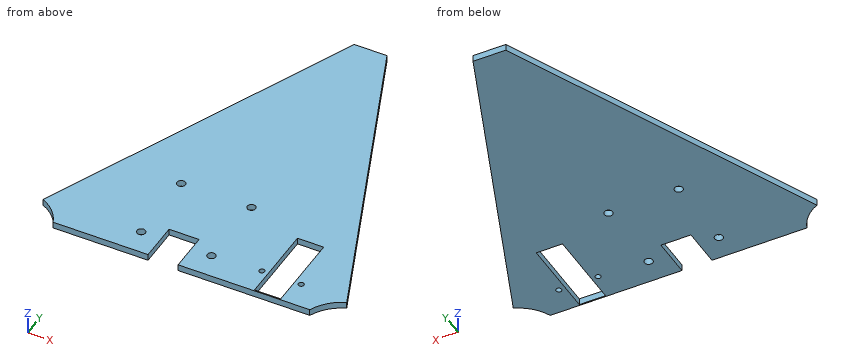
from build123d import *

# Parameters (mm, degrees)
BOSS_EXTRUDE1_DEPTH     = 7.62
SKETCH5_R               = 15.875
CUT_EXTRUDE2_DEPTH      = 50.8
SKETCH6_R               = 15.875
CUT_EXTRUDE3_DEPTH      = 50.8
CUT_EXTRUDE4_DEPTH      = 444.557362906
CUT_EXTRUDE4_DEPTH_BACK = 7.62
CUT_EXTRUDE6_REACH      = 445.557
SKETCH9_R               = 4.826
SKETCH10_W              = 30.48
SKETCH10_H              = 114.3
CUT_EXTRUDE12_DEPTH     = 25.4
CUT_EXTRUDE14_REACH     = 445.557
SKETCH14_R              = 50.8
CUT_EXTRUDE15_REACH     = 445.557
SKETCH15_R              = 50.8
SKETCH16_W              = 30.48
SKETCH16_H              = 20.32
BOSS_EXTRUDE2_DEPTH     = 7.62
CUT_EXTRUDE16_REACH     = 433.743
SKETCH17_R              = 3.175
CUT_EXTRUDE17_START     = -7.62
SKETCH18_W              = 300.609514784
SKETCH18_H              = 19.05
CUT_EXTRUDE17_DEPTH     = 7.62
CUT_EXTRUDE18_REACH     = 433.743
SKETCH19_R              = 4.826


with BuildPart() as part:
    # Sketch2 → Boss-Extrude1 (new body)
    with BuildSketch(Plane.XY):
        Polygon((-189.740054039, 245.383385713), (-375.90852523, -170.414614287), (16.77547477, -170.414614287), (-151.640054039, 245.383385713), align=None)
    extrude(amount=BOSS_EXTRUDE1_DEPTH)

    # Sketch5 → Cut-Extrude2 (cut)
    with BuildSketch(Plane(origin=(0, 0, 0), x_dir=(-1, 0, 0), z_dir=(0, 0, -1))):
        with Locations((375.90852523, -170.414614287)):
            Circle(SKETCH5_R)
    extrude(amount=-CUT_EXTRUDE2_DEPTH, mode=Mode.SUBTRACT)

    # Sketch6 → Cut-Extrude3 (cut)
    with BuildSketch(Plane(origin=(0, 0, 0), x_dir=(-1, 0, 0), z_dir=(0, 0, -1))):
        with Locations((-16.77547477, -170.414614287)):
            Circle(SKETCH6_R)
    extrude(amount=-CUT_EXTRUDE3_DEPTH, mode=Mode.SUBTRACT)

    # Sketch8 → Cut-Extrude4 (cut, two sides: drawn at the far end of the back side and taken through both)
    with BuildSketch(Plane(origin=(0, 0, 0), x_dir=(-1, 0, 0), z_dir=(0, 0, -1)).offset(-CUT_EXTRUDE4_DEPTH_BACK)):
        Polygon((218.448947474, -1130.046710402), (218.448947474, -170.414614287), (218.448947474, -105.390614287), (183.523947474, -105.390614287), (183.523947474, -170.414614287), (183.523947474, -1130.046710402), (183.523947474, -3049.310902633), (218.448947474, -3049.310902633), align=None)
    extrude(amount=CUT_EXTRUDE4_DEPTH + CUT_EXTRUDE4_DEPTH_BACK, mode=Mode.SUBTRACT)

    # Sketch9 → Cut-Extrude6 (cut, up to next)
    with BuildSketch(Plane(origin=(0, 0, 0), x_dir=(-1, 0, 0), z_dir=(0, 0, -1)), mode=Mode.PRIVATE) as cut_extrude6_sk1:
        with Locations((160.155947474, -122.408614287)):
            Circle(SKETCH9_R)
    cut_extrude6_tool1 = extrude(cut_extrude6_sk1.sketch, amount=-CUT_EXTRUDE6_REACH, mode=Mode.PRIVATE) & part.part
    # Sketch9 → Cut-Extrude6 (cut, up to next)
    with BuildSketch(Plane(origin=(0, 0, 0), x_dir=(-1, 0, 0), z_dir=(0, 0, -1)), mode=Mode.PRIVATE) as cut_extrude6_sk2:
        with Locations((241.816947474, -122.408614287)):
            Circle(SKETCH9_R)
    cut_extrude6_tool2 = extrude(cut_extrude6_sk2.sketch, amount=-CUT_EXTRUDE6_REACH, mode=Mode.PRIVATE) & part.part
    add(cut_extrude6_tool1.solids().sort_by_distance((-160.155947, -122.408614, 0))[0], mode=Mode.SUBTRACT)
    add(cut_extrude6_tool2.solids().sort_by_distance((-241.816947, -122.408614, 0))[0], mode=Mode.SUBTRACT)

    # Sketch10 → Cut-Extrude12 (cut)
    with BuildSketch(Plane(origin=(0, 0, 0), x_dir=(-1, 0, 0), z_dir=(0, 0, -1))):
        with Locations((80.066257047, -113.264614287)):
            Rectangle(SKETCH10_W, SKETCH10_H)
    extrude(amount=-CUT_EXTRUDE12_DEPTH, mode=Mode.SUBTRACT)

    # Sketch14 → Cut-Extrude14 (cut, up to next)
    with BuildSketch(Plane(origin=(0, 0, 0), x_dir=(-1, 0, 0), z_dir=(0, 0, -1)), mode=Mode.PRIVATE) as cut_extrude14_sk1:
        with Locations((-16.77547477, -170.414614287)):
            Circle(SKETCH14_R)
    cut_extrude14_tool1 = extrude(cut_extrude14_sk1.sketch, amount=-CUT_EXTRUDE14_REACH, mode=Mode.PRIVATE) & part.part
    add(cut_extrude14_tool1.solids().sort_by_distance((16.775475, -170.414614, 0))[0], mode=Mode.SUBTRACT)

    # Sketch15 → Cut-Extrude15 (cut, up to next)
    with BuildSketch(Plane(origin=(0, 0, 0), x_dir=(-1, 0, 0), z_dir=(0, 0, -1)), mode=Mode.PRIVATE) as cut_extrude15_sk1:
        with Locations((375.90852523, -170.414614287)):
            Circle(SKETCH15_R)
    cut_extrude15_tool1 = extrude(cut_extrude15_sk1.sketch, amount=-CUT_EXTRUDE15_REACH, mode=Mode.PRIVATE) & part.part
    add(cut_extrude15_tool1.solids().sort_by_distance((-375.908525, -170.414614, 0))[0], mode=Mode.SUBTRACT)

    # Sketch16 → Boss-Extrude2 (add)
    with BuildSketch(Plane(origin=(0, 0, 0), x_dir=(-1, 0, 0), z_dir=(0, 0, -1))):
        with Locations((80.066257047, -160.254614287)):
            Rectangle(SKETCH16_W, SKETCH16_H)
    extrude(amount=-BOSS_EXTRUDE2_DEPTH)

    # Sketch17 → Cut-Extrude16 (cut, up to next)
    with BuildSketch(Plane(origin=(0, 0, 0), x_dir=(-1, 0, 0), z_dir=(0, 0, -1)), mode=Mode.PRIVATE) as cut_extrude16_sk1:
        with Locations((57.206257047, -119.614614287)):
            Circle(SKETCH17_R)
    cut_extrude16_tool1 = extrude(cut_extrude16_sk1.sketch, amount=-CUT_EXTRUDE16_REACH, mode=Mode.PRIVATE) & part.part
    # Sketch17 → Cut-Extrude16 (cut, up to next)
    with BuildSketch(Plane(origin=(0, 0, 0), x_dir=(-1, 0, 0), z_dir=(0, 0, -1)), mode=Mode.PRIVATE) as cut_extrude16_sk2:
        with Locations((102.926257047, -119.614614287)):
            Circle(SKETCH17_R)
    cut_extrude16_tool2 = extrude(cut_extrude16_sk2.sketch, amount=-CUT_EXTRUDE16_REACH, mode=Mode.PRIVATE) & part.part
    add(cut_extrude16_tool1.solids().sort_by_distance((-57.206257, -119.614614, 0))[0], mode=Mode.SUBTRACT)
    add(cut_extrude16_tool2.solids().sort_by_distance((-102.926257, -119.614614, 0))[0], mode=Mode.SUBTRACT)

    # Sketch18 → Cut-Extrude17 (cut)
    with BuildSketch(Plane(origin=(0, 0, 0), x_dir=(-1, 0, 0), z_dir=(0, 0, -1)).offset(CUT_EXTRUDE17_START)):
        with Locations((180.749872138, -160.889614287)):
            Rectangle(SKETCH18_W, SKETCH18_H)
    extrude(amount=CUT_EXTRUDE17_DEPTH, mode=Mode.SUBTRACT)

    # Sketch19 → Cut-Extrude18 (cut, up to next)
    with BuildSketch(Plane(origin=(0, 0, 0), x_dir=(-1, 0, 0), z_dir=(0, 0, -1)), mode=Mode.PRIVATE) as cut_extrude18_sk1:
        with Locations((241.816947474, -34.778614287)):
            Circle(SKETCH19_R)
    cut_extrude18_tool1 = extrude(cut_extrude18_sk1.sketch, amount=-CUT_EXTRUDE18_REACH, mode=Mode.PRIVATE) & part.part
    # Sketch19 → Cut-Extrude18 (cut, up to next)
    with BuildSketch(Plane(origin=(0, 0, 0), x_dir=(-1, 0, 0), z_dir=(0, 0, -1)), mode=Mode.PRIVATE) as cut_extrude18_sk2:
        with Locations((160.155947474, -34.778614287)):
            Circle(SKETCH19_R)
    cut_extrude18_tool2 = extrude(cut_extrude18_sk2.sketch, amount=-CUT_EXTRUDE18_REACH, mode=Mode.PRIVATE) & part.part
    add(cut_extrude18_tool1.solids().sort_by_distance((-241.816947, -34.778614, 0))[0], mode=Mode.SUBTRACT)
    add(cut_extrude18_tool2.solids().sort_by_distance((-160.155947, -34.778614, 0))[0], mode=Mode.SUBTRACT)


solid = part.part
Work out the finished part from the listing and answer in its coordinate system (mm). Round coordinates to 2 decimals unless told otherwise and drop trailing zeros. Write each loop counter-clockwise with the first axis right and the second up, starting at its lowest first coordinate (ties: lowest second). Pieces come first, ordered by that corner, then holes. Notation, with made-up numbers: M -32,15 L 6,15 A20 ccw 6,42 Z; hole C 37.5,-16 d3. An arc over 180 degrees is marked long. Use a Markdown table: item, result.
1) Flat-ended cylindrical pins translate along their axes: pin 1 (2 mm diameter, centred on y = 14.5, z = 3, fed in from +X); pin 2 (1 mm diameter, centred on x = -126.5, y = -79.5, fed in from -Z); pin 3 (4 mm diameter, centred on y = -138, z = 5, fed in from -X); pin 4 (2.5 mm diameter, centred on x = -124, z = 4.5, fed in from -Y). Find the tip coordinate at first contact, or state that the pin passes through.
Taken from the geometry:
| item | result |
|---|---|
| pin 1 | stops at x = -57.72 |
| pin 2 | stops at z = 0 |
| pin 3 | stops at x = -338.54 |
| pin 4 | stops at y = -151.36 |
2) The part is cut by section B-B on z = 3. Give the vertices of the cut face in (x, y) (3 decimals), plus the area to 3 significant figures.
Taken from the geometry:
| item | result |
|---|---|
| outline | M -355.149,-124.05 A50.8 cw -328.816,-151.365 L -218.449,-151.365 L -218.449,-105.391 L -183.524,-105.391 L -183.524,-151.365 L -30.445,-151.365 L -30.445,-151.683 A50.8 cw -2.296,-123.33 L -151.64,245.383 L -189.74,245.383 Z; hole C -241.817,-122.409 d9.652; hole C -241.817,-34.779 d9.652; hole C -160.156,-122.409 d9.652; hole C -160.156,-34.779 d9.652; hole C -102.926,-119.615 d6.35; hole M -95.306,-150.095 L -64.826,-150.095 L -64.826,-56.115 L -95.306,-56.115 Z; hole C -57.206,-119.615 d6.35 |
| area | 76,100 mm2 |
3) The part is cut by section A-A on x = -81. Give the vertices of the cut face in (y, z).
Taken from the geometry:
| item | result |
|---|---|
| outline | M -151.36,0 L -150.09,0 L -150.09,7.62 L -151.36,7.62 Z; M -56.11,0 L 70.98,0 L 70.98,7.62 L -56.11,7.62 Z |
4) Consider line 1 (X direction, y = -124.5, z = 6.25); line 2 (X direction, y = -131, z = 1.75); line 3 (X direction, y = -32, z = 7). Determine where each line is inside the solid, lowest interval first. Write a range as [from, to].
Taken from the geometry:
| item | result |
|---|---|
| line 1 | x = [-354.17, -246.17], [-237.47, -218.45], [-183.52, -164.51], [-155.81, -95.31], [-64.83, -4.96] |
| line 2 | x = [-343.86, -218.45], [-183.52, -95.31], [-64.83, -15.27] |
| line 3 | x = [-313.94, -245.76], [-237.87, -164.1], [-156.21, -39.29] |
5) The part is cut by section C-C on y = -4.5. Give the vertices of the cut face in (x, z).
Taken from the geometry:
| item | result |
|---|---|
| outline | M -301.62,0 L -50.43,0 L -50.43,7.62 L -301.62,7.62 Z |
6) The part is cut by section D-D on x = -291. Give the vertices of the cut face in (y, z), plus the area to 3 significant figures.
Taken from the geometry:
| item | result |
|---|---|
| outline | M -151.36,0 L 19.22,0 L 19.22,7.62 L -151.36,7.62 Z |
| area | 1,300 mm2 |
